The listing builds one solid part. Answer for the finished solid, in the listing's coordinates (mm). A direction names the side the tool comes from. Round coordinates to 2 decimals unless told otherwise and drop trailing zeros. Write each loop counter-clockwise with the first axis right and the second up, starting at its lowest first coordinate (ties: lowest second). Pieces come first, ordered by that corner, then holes. Notation, with made-up numbers: (-16.5, 18.25) - (1.5, 18.25) arc R27 ccw to (1.5, 41.25) - close; hole circle Ø1 at (62, 79). An arc over 180 degrees is marked (long way). Return JSON: item names as keys, results as strings. Group by question number.
(1) Determine the mould class of faces 1 (the flat face through (57, 18, 32)), 2 (the flat face through (57, 18, 29)), 3 (the flat face through (111, 56, 29)), 4 (the flat face through (-3, 31, 16)) for opening direction X: +X half, -X half, draft (parallel to the pull), parting line (faces both ways), or undercut.
(2) Each of these flat-tipped pins is pushed along its axis until it touches: pin 1 (2 mm diameter, centred on y = 0.5, z = 28, fed in from -X); pin 2 (0.9 mm diameter, centred on x = 4, y = 4, fed in from -Z); pin 3 (11 mm diameter, centred on x = 106.5, z = 8, fed in from -Y); pin 4 (1.5 mm diameter, centred on x = 111, y = 57, fed in from -Z). Where does it stop, or does it pass through?
(3) Find the intervals of material crossed by line 1 along Y through (x, z) = (111.2, 20.25); line 2 along Y through (x, z) = (24, 24.5); line 3 along X through (y, z) = (-16, 2), in increasing order. Write a range as [from, to].
(4) Section C-C, the plane x = 111.2 is taken. Write down the section's boundary in (y, z).
(5) Section D-D, the plane y = -10 is taken. Write down the section's boundary in (x, z), then the cut area to 3 significant figures.
(6) Section A-A, the plane y = 13 is taken. Write down the section's boundary in (x, z), then the cut area to 3 significant figures.
(7) Which of the six approach directions +Z, -Z, +X, -X, +Y, -Y give full straight-line access (tool end or side, diameter ignored) to faces 5 (the flat face through (51.1, -27, 3)), 6 (the cylindrical face through (16.341, -26.997, 16.224)), 7 (the flat face through (0, 30, 14))?
(8) Section B-B, the plane z = 25.5 is taken. Give the number of separate pieces and of enclosed holes in the cut face, then the cut area to 3 significant figures.
```python
from build123d import *

# Parameters (mm, degrees)
DODANIE_WYCI_GNI_CIE1_DEPTH = 29
DODANIE_WYCI_GNI_CIE2_DEPTH = 3
SZKIC3_R                    = 3
SZKIC3_R_2                  = 1.5
DODANIE_WYCI_GNI_CIE3_DEPTH = 22
SZKIC5_W                    = 13
SZKIC5_H                    = 6
WYTNIJ_WYCI_GNI_CIE1_DEPTH  = 7
ZAOKR_GLENIE1_R             = 4
ZAOKR_GLENIE2_R             = 4


with BuildPart() as part:
    # Szkic1 → Dodanie-wyciągnięcie1 (new body)
    with BuildSketch(Plane.XY):
        Polygon((-1.456531899, 63.2), (118.2, 63.2), (118.2, -3), (100, -3), (100, -28.2), (15.2, -28.2), (15.2, -3), (-3, -3), (-3, 63.2), align=None)
        Polygon((0, 0), (0, 60.2), (115.2, 60.2), (115.2, 0), (97, 0), (97, -25.2), (18.2, -25.2), (18.2, 0), align=None, mode=Mode.SUBTRACT)
    extrude(amount=DODANIE_WYCI_GNI_CIE1_DEPTH)

    # Szkic2 → Dodanie-wyciągnięcie2 (add)
    with BuildSketch(Plane.XY.offset(29)):
        Polygon((-3, 63.2), (-3, -3), (15.2, -3), (15.2, -28.2), (100, -28.2), (100, -3), (118.2, -3), (118.2, 63.2), align=None)
    extrude(amount=DODANIE_WYCI_GNI_CIE2_DEPTH)

    # Szkic3 → Dodanie-wyciągnięcie3 (add)
    # profile 1 of 4: a face of its own
    with BuildSketch(Plane(origin=(0, 0, 29), x_dir=(-1, 0, 0), z_dir=(0, 0, -1))):
        with Locations(Location((-111.2, 4, 0), (0, 0, 180))):
            Circle(SZKIC3_R)
        with Locations((-111.2, 4)):
            Circle(SZKIC3_R_2, mode=Mode.SUBTRACT)
    # profile 2 of 4: a face of its own
    with BuildSketch(Plane(origin=(0, 0, 29), x_dir=(-1, 0, 0), z_dir=(0, 0, -1))):
        with Locations(Location((-111.2, 56.2, 0), (0, 0, 180))):
            Circle(SZKIC3_R)
        with Locations((-111.2, 56.2)):
            Circle(SZKIC3_R_2, mode=Mode.SUBTRACT)
    # profile 3 of 4: a face of its own
    with BuildSketch(Plane(origin=(0, 0, 29), x_dir=(-1, 0, 0), z_dir=(0, 0, -1))):
        with Locations(Location((-3.901278793, 56.103657268, 0), (0, 0, 180))):
            Circle(SZKIC3_R)
        with Locations((-3.901278793, 56.103657268)):
            Circle(SZKIC3_R_2, mode=Mode.SUBTRACT)
    # profile 4 of 4: a face of its own
    with BuildSketch(Plane(origin=(0, 0, 29), x_dir=(-1, 0, 0), z_dir=(0, 0, -1))):
        with Locations(Location((-4.096342732, 3.901278793, 0), (0, 0, 180))):
            Circle(SZKIC3_R)
        with Locations((-4.096342732, 3.901278793)):
            Circle(SZKIC3_R_2, mode=Mode.SUBTRACT)
    extrude(amount=DODANIE_WYCI_GNI_CIE3_DEPTH)

    # Szkic5 → Wytnij-wyciągnięcie1 (cut)
    with BuildSketch(Plane(origin=(0, 0, 0), x_dir=(-1, 0, 0), z_dir=(0, 0, -1))):
        with Locations((-57.6, -25.2)):
            Rectangle(SZKIC5_W, SZKIC5_H)
    extrude(amount=-WYTNIJ_WYCI_GNI_CIE1_DEPTH, mode=Mode.SUBTRACT)

    # Zaokrąglenie1
    zaokr_glenie1_edges = [part.edges().sort_by_distance(p)[0] for p in [
        (118.2, 63.2, 16),
        (118.2, -3, 16),
        (100, -28.2, 16),
        (15.2, -28.2, 16),
        (-3, -3, 16),
        (-3, 63.2, 16),
    ]]
    fillet(zaokr_glenie1_edges, radius=ZAOKR_GLENIE1_R)

    # Zaokrąglenie2
    zaokr_glenie2_edges = [part.edges().sort_by_distance(p)[0] for p in [
        (100, -3, 16),
        (15.2, -3, 16),
    ]]
    fillet(zaokr_glenie2_edges, radius=ZAOKR_GLENIE2_R)


solid = part.part
```
Working result:
{
 "1": {"face 1": "draft", "face 2": "undercut", "face 3": "undercut", "face 4": "-X half"},
 "2": {"pin 1": "stops at x = -3", "pin 2": "stops at z = 29", "pin 3": "stops at y = -4.35", "pin 4": "stops at z = 7"},
 "3": {"line 1": "y = [-3, 0], [1, 2.5], [5.5, 7], [53.2, 54.7], [57.7, 59.2], [60.2, 63.2]", "line 2": "y = [-28.2, -25.2], [60.2, 63.2]", "line 3": "x = [15.2, 18.2], [97, 100]"},
 "4": {"outline": "(-3, 0) - (0, 0) - (0, 29) - (1, 29) - (1, 7) - (2.5, 7) - (2.5, 29) - (5.5, 29) - (5.5, 7) - (7, 7) - (7, 29) - (53.2, 29) - (53.2, 7) - (54.7, 7) - (54.7, 29) - (57.7, 29) - (57.7, 7) - (59.2, 7) - (59.2, 29) - (60.2, 29) - (60.2, 0) - (63.2, 0) - (63.2, 32) - (-3, 32) - close"},
 "5": {"outline": "(15.2, 0) - (18.2, 0) - (18.2, 29) - (97, 29) - (97, 0) - (100, 0) - (100, 32) - (15.2, 32) - close", "area": "428 mm^2"},
 "6": {"outline": "(-3, 0) - (0, 0) - (0, 29) - (115.2, 29) - (115.2, 0) - (118.2, 0) - (118.2, 32) - (-3, 32) - close", "area": "538 mm^2"},
 "7": {"face 5": "-Z, -Y", "face 6": "+Z, -Z, -X, -Y", "face 7": "-Z"},
 "8": {"separate pieces": "5", "enclosed holes": "5", "area": "1,310 mm^2"}
}
